Can you work these out from the drawing? Everything is in mm from the part's minimum corner. A direction names the side the tool comes from. Coordinates: 2 decimals unless noted, no trailing zeros. Write each loop counter-clockwise with the first axis right and the second up, starting at its lowest first coordinate (ties: lowest second). Pieces come first, ordered by that corner, then holes. Notation, with made-up numbers: M 46.5,-28 L 102.5,-28 A27 ccw 102.5,2 Z; hole C 88,27.5 d9. An arc over 180 degrees is marked long. Write each question's results on one line, items separated by ' | '. Start each with the question number.
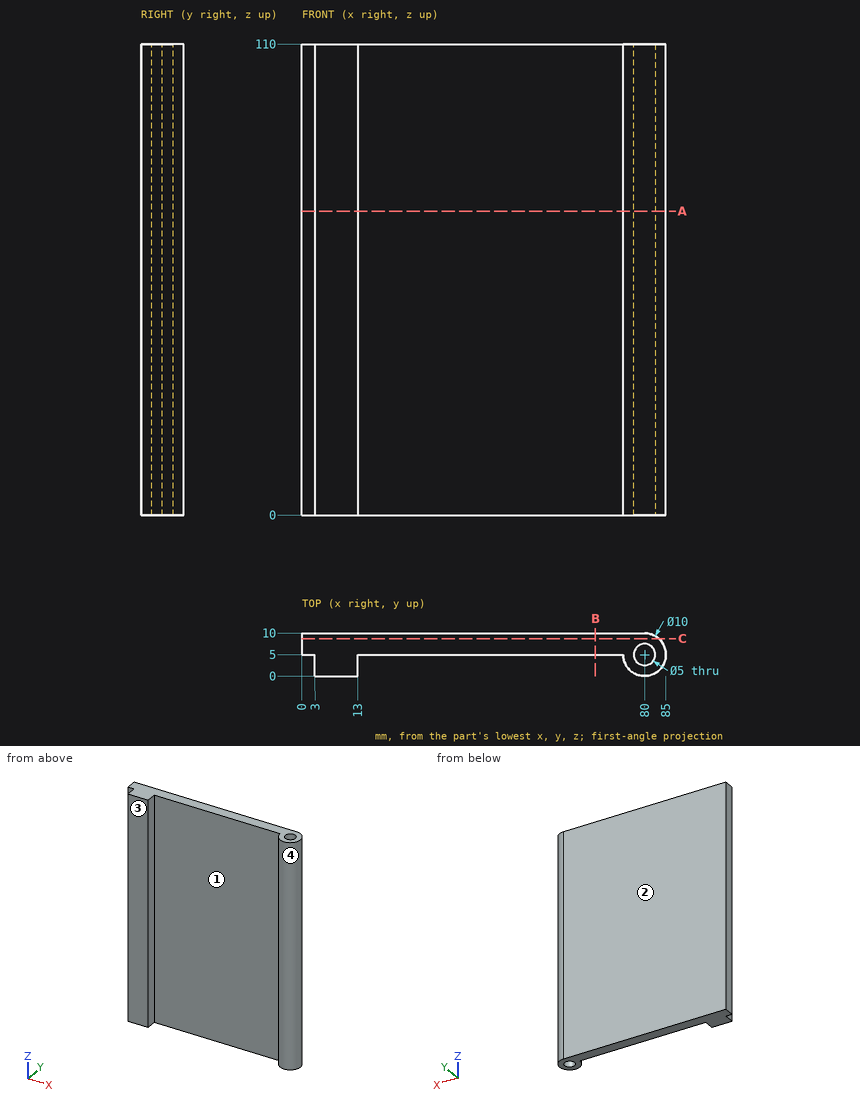
1) For the marked faces 1 and 2, which set-ups out of +Z, -Z, +X, -X, +Y, -Y let a thin tool reach every point of the face, with its end or its side?
2) Please list where these lines run through material, in increasing order: line 1 (Y direction, x = 80, z = 51); line 2 (X direction, y = 3, z = 96); line 3 (Y direction, x = 36.5, z = 64.5). Write a range as [from, to].
3) For pin 1 Ø1 at (y, z) = (3.5, 18.5) entering from +X; pin 2 Ø1.5 at (x, z) = (2, 78) entering from -Y; pin 3 Ø2 at (y, z) = (1, 73) entering from +X, each with a flat end and sliding along its axis, tell me the tip position at first contact or that it passes through.
4) I want a section at A-A, the plane z = 71. Write out the boundary of the cut face in (x, y), then the cut area to 3 significant figures.
5) I want a section at C-C, the plane y = 8.75. Write out the boundary of the cut face in (x, z), then the cut area to 3 significant figures.
6) I want a section at B-B, the plane x = 68.5. Write out the boundary of the cut face in (y, z), then the cut area to 3 significant figures.
7) We'd pull the mould along X, two halves only. Please class the marked faces 3 and 4: pulls with the +X half, pulls with the -X half, needs draft (parallel to the pull), parting line crosses it, or undercut.
Output:
1) face 1: +Z, -Z, -Y | face 2: +Z, -Z, +X, -X, +Y
2) line 1: y = [0, 2.5], [7.5, 10] | line 2: x = [3, 13], [75.42, 78.5], [81.5, 84.58] | line 3: y = [5, 10]
3) pin 1: stops at x = 84.9 | pin 2: stops at y = 5 | pin 3: stops at x = 84
4) outline: M 0,5 L 3,5 L 3,0 L 13,0 L 13,5 L 75,5 A5 ccw long 80,10 L 0,10 Z; hole C 80,5 d5 | area: 489 mm2
5) outline: M 0,0 L 83.31,0 L 83.31,110 L 0,110 Z | area: 9,160 mm2
6) outline: M 5,0 L 10,0 L 10,110 L 5,110 Z | area: 550 mm2
7) face 3: needs draft | face 4: undercut
